from build123d import *

# Parameters (mm, degrees)
F0_R     = 19.05
F1_DEPTH = 38.1
F2_DEPTH = 25.4
F3_DEPTH = 31.75


with BuildPart() as f1:
    # F0 (on Top) → F1 (new body)
    with BuildSketch(Plane.XY):
        with BuildLine():
            ThreePointArc((2.581912, -25.268433), (18.851268, -17.023211), (25.4, 0))
            ThreePointArc((25.4, 0), (18.833823, 17.042509), (2.530148, 25.273669))
            ThreePointArc((2.530148, 25.273669), (-25.399987, -0.026014), (2.581912, -25.268433))
        make_face()
        Circle(F0_R, mode=Mode.SUBTRACT)
    extrude(amount=F1_DEPTH)

    # F0 (on Top) → F2 (join)
    with BuildSketch(Plane.XY):
        with BuildLine():
            ThreePointArc((2.530148, 25.273669), (18.833823, 17.042509), (25.4, 0))
            ThreePointArc((25.4, 0), (18.851268, -17.023211), (2.581912, -25.268433))
            Line((2.581912, -25.268433), (127.494344, -12.504961))
            ThreePointArc((127.494344, -12.504961), (117.691782, -9.296378), (113.503388, 0.129256))
            ThreePointArc((113.503388, 0.129256), (117.682133, 9.546167), (127.468462, 12.76609))
            Line((127.468462, 12.76609), (2.530148, 25.273669))
        make_face()
        with BuildLine():
            ThreePointArc((37.3036, -6.220744), (30.953388, 0.12915), (37.303388, 6.479256))
            Line((37.303388, 6.479256), (88.103176, 6.480948))
            ThreePointArc((88.103176, 6.480948), (94.453176, 0.131054), (88.103388, -6.219052))
            Line((88.103388, -6.219052), (37.3036, -6.220744))
        make_face(mode=Mode.SUBTRACT)
    extrude(amount=F2_DEPTH)

    # F0 (on Top) → F3 (join)
    with BuildSketch(Plane.XY):
        with BuildLine():
            ThreePointArc((138.903388, 0.129256), (135.620299, 8.65051), (127.468462, 12.76609))
            ThreePointArc((127.468462, 12.76609), (117.682133, 9.546167), (113.503388, 0.129256))
            ThreePointArc((113.503388, 0.129256), (117.691782, -9.296378), (127.494344, -12.504961))
            ThreePointArc((127.494344, -12.504961), (135.629022, -8.38235), (138.903388, 0.129256))
        make_face()
        with BuildLine():
            ThreePointArc((132.553388, 0.129256), (126.203388, -6.220744), (119.853388, 0.129256))
            ThreePointArc((119.853388, 0.129256), (126.203388, 6.479256), (132.553388, 0.129256))
        make_face(mode=Mode.SUBTRACT)
    extrude(amount=F3_DEPTH)


solid = f1.part
Verification items for the finished model (mm, model axes). A direction names the side the tool comes from. Coordinates: 2 decimals unless noted, no trailing zeros. Order: outer loops, then holes, each group sorted by start corner. A loop starts at its lowest first (then second) coordinate and runs counter-clockwise, first axis right, second up. Notation, with made-up numbers: M -25,-27 L -10,-27 A20 cw -10,-6 Z; hole C -14,83 d2. An arc over 180 degrees is marked long. Return JSON: item names as keys, results as strings.
1) Cross-section at D-D, the plane x = 43. Record the boundary of the cut face in (y, z), and give its area (3 significant figures).
Answer list:
{"outline": "M -21.14,0 L -6.22,0 L -6.22,25.4 L -21.14,25.4 Z; M 6.48,0 L 21.22,0 L 21.22,25.4 L 6.48,25.4 Z", "area": "753 mm2"}
2) Cross-section at B-B, the plane z = 19.5. Record the boundary of the cut face in (x, y), and give its area (3 significant figures).
Answer list:
{"outline": "M 2.53,25.27 A25.4 ccw long 2.58,-25.27 L 127.49,-12.5 A12.7 ccw 138.9,0.13 A12.7 ccw 127.47,12.77 Z; hole C 0,0 d38.1; hole M 37.3,-6.22 L 88.1,-6.22 A6.35 ccw 88.1,6.48 L 37.3,6.48 A6.35 ccw Z; hole C 126.2,0.13 d12.7", "area": "4,060 mm2"}
3) Gauge pin test, flat ends, axial feed: pin 1 (8 mm diameter, centred on x = 26, z = 13, fed in from +Y); pin 2 (12.5 mm diameter, centred on x = 126.5, y = -1.5, fed in from +Z); pin 3 (6 mm diameter, centred on y = -14.5, z = 7.5, fed in from -X). Record the tip position at first contact, or that the pin passes through.
Answer list:
{"pin 1": "y = 23.32", "pin 2": "z = 31.75", "pin 3": "x = -22.65"}
4) Cross-section at A-A, the plane x = 0. Record the boundary of the cut face in (y, z).
Answer list:
{"outline": "M -25.4,0 L -19.05,0 L -19.05,38.1 L -25.4,38.1 Z; M 19.05,0 L 25.4,0 L 25.4,38.1 L 19.05,38.1 Z"}
5) Release check for a two-part mould opening along Y. For faces 1 (the flat face through (64, -11, 25.4)), 2 (the cylindrical face through (30.955, -0.01, 12.522)), 3 (the flat face through (65.874, 18.932, 12.522)) record: +Y half, -Y half, draft (parallel to the pull), parting line (faces both ways), or undercut.
Answer list:
{"face 1": "draft", "face 2": "undercut", "face 3": "+Y half"}
6) Access from +Z, -Z, +X, -X, +Y, -Y to the whole of each face (thin tool, end or side, straight path). Record for faces 4 (the cylindrical face through (94.45, 0.27, 12.52)), 5 (the flat face through (64.164, -18.976, 12.522)), 6 (the flat face through (129, 6, 31.75)).
Answer list:
{"face 4": "+Z, -Z", "face 5": "+Z, -Z, +X, -Y", "face 6": "+Z, +X, +Y, -Y"}
7) Cross-section at C-C, the plane y = -8. Record the boundary of the cut face in (x, z).
Answer list:
{"outline": "M -24.11,0 L -17.29,0 L -17.29,38.1 L -24.11,38.1 Z; M 17.29,0 L 135.96,0 L 135.96,31.75 L 116.45,31.75 L 116.45,25.4 L 24.11,25.4 L 24.11,38.1 L 17.29,38.1 Z"}
8) Thickness scan on L1, parallel to X at y = 8, z = 31; L2, parallel to X at y = -5, z = 27; L3, parallel to Y at x = 0, z = 24. Record the ranges inside material, lowest first. Write a range as [from, to].
Answer list:
{"L1": "[-24.11, -17.29], [17.29, 24.11], [116.24, 136.17]", "L2": "[-24.9, -18.38], [18.38, 24.9], [114.59, 122.46], [129.95, 137.82]", "L3": "[-25.4, -19.05], [19.05, 25.4]"}
